Design review of the part built by this model. Coordinates are the model's own, in mm. Face numbers are marked on the shaded views. Coordinates: 2 decimals unless noted, no trailing zeros. Loops run counter-clockwise (first coordinate to the right, second up) from the corner with the lowest first, then second, coordinate; pieces in that order, holes last. Notation, with made-up numbers: (54.25, 68) -> (61.25, 68) arc R18 cw to (61.25, 98) -> close; hole circle Ø3 at (80, 89.5). An arc over 180 degrees is marked (long way). Use CSV: the item, a comma, the result in double quotes.
```python
from build123d import *

# Parameters (mm, degrees)
EXTRUDE_1_DEPTH             = 20
SKETCH_2_R                  = 15
CUT_EXTRUDE_1_DEPTH         = 21
CUT_EXTRUDE_2_DEPTH         = 5
HOLE_WIZARD_M6_1_D          = 5
HOLE_WIZARD_M6_1_DEPTH      = 15
HOLE_WIZARD_M6_1_TIP        = 1.502151548
HOLE_WIZARD_M6_2_AT_2_COUNT = 2
HOLE_WIZARD_M6_2_AT_2_PITCH = 40
MM_1_D                      = 12
MM_1_DEPTH                  = 2
MM_1_TIP                    = 3.605163714
SKETCH_19_W                 = 298.256507651
SKETCH_19_H                 = 73.483487392
SKETCH_19_W_2               = 296.09522861
CUT_EXTRUDE_3_DEPTH         = 21


with BuildPart() as part:
    # 草图1 → 凸台-拉伸1 (new body)
    with BuildSketch(Plane.XY):
        Polygon((-580, 85), (-600, 65), (-600, -65), (-580, -85), (580, -85), (600, -65), (600, 65), (580, 85), align=None)
    extrude(amount=EXTRUDE_1_DEPTH)

    # 草图2 → 切除-拉伸1 (cut, through all)
    with BuildSketch(Plane.XY.offset(20)):
        with Locations((540, 0)):
            Circle(SKETCH_2_R)
    extrude(amount=-CUT_EXTRUDE_1_DEPTH, mode=Mode.SUBTRACT)

    # 草图3 → 切除-拉伸2 (cut)
    with BuildSketch(Plane.XY.offset(20)):
        with BuildLine():
            Line((-800, -60), (-405, -60))
            ThreePointArc((-405, -60), (-401.464466094, -58.535533906), (-400, -55))
            Line((-400, -55), (-400, 55))
            ThreePointArc((-400, 55), (-401.464466094, 58.535533906), (-405, 60))
            Line((-405, 60), (-800, 60))
            Line((-800, 60), (-800, -60))
        make_face()
    extrude(amount=-CUT_EXTRUDE_2_DEPTH, mode=Mode.SUBTRACT)

    # M6 螺纹孔1
    with Locations(Plane(origin=(-390, 25, 20), x_dir=(1, 0, 0), z_dir=(0, 0, 1))):
        with Locations((0, 0), (0, -50)):
            Hole(HOLE_WIZARD_M6_1_D / 2, depth=HOLE_WIZARD_M6_1_DEPTH)
            with Locations((0, 0, -(HOLE_WIZARD_M6_1_DEPTH + HOLE_WIZARD_M6_1_TIP / 2))):  # 118° drill point
                Cone(0, HOLE_WIZARD_M6_1_D / 2, HOLE_WIZARD_M6_1_TIP, mode=Mode.SUBTRACT)

    # 草图16 → M6 螺纹孔2 (revolve, cut)
    with BuildSketch(Plane(origin=(400, 60, 20), x_dir=(0, -1, 0), z_dir=(1, 0, 0))):
        Polygon((0, 0), (0, 16.502151548), (2.5, 15), (2.5, 0), align=None)
    hole_wizard_m6_2 = revolve(axis=Axis((400, 60, 26.35), (0, 0, -1)), mode=Mode.SUBTRACT)

    # M6 螺纹孔2 at 2: M6 螺纹孔2 ×2
    with Locations(*[(i * HOLE_WIZARD_M6_2_AT_2_PITCH, 0, 0) for i in range(1, HOLE_WIZARD_M6_2_AT_2_COUNT)]):
        add(hole_wizard_m6_2, mode=Mode.SUBTRACT)

    # 镜向2: M6 螺纹孔2 across plane
    add(hole_wizard_m6_2.mirror(Plane.ZX), mode=Mode.SUBTRACT)

    # 镜向2 copy 1 sketch → 镜向2 copy 1 (revolve, cut)
    with BuildSketch(Plane(origin=(440, -60, 20), x_dir=(0, 1, 0), z_dir=(1, 0, 0))):
        Polygon((0, 0), (0, -16.502151548), (2.5, -15), (2.5, 0), align=None)
    revolve(axis=Axis((440, -60, 26.35), (0, 0, 1)), mode=Mode.SUBTRACT)

    # 大小mm 暗销孔1
    with Locations(Plane(origin=(0, 0, 0), x_dir=(-1, 0, 0), z_dir=(0, 0, -1))):
        with Locations((-250, 65), (250, 65), (250, -65), (-250, -65)):
            Hole(MM_1_D / 2, depth=MM_1_DEPTH)
            with Locations((0, 0, -(MM_1_DEPTH + MM_1_TIP / 2))):  # 118° drill point
                Cone(0, MM_1_D / 2, MM_1_TIP, mode=Mode.SUBTRACT)

    # 草图19 → 切除-拉伸3 (cut, through all)
    with BuildSketch(Plane.XY.offset(20)):
        with Locations((-182.687664533, 0)):
            Rectangle(SKETCH_19_W, SKETCH_19_H)
        with Locations((286.309887354, 0)):
            Rectangle(SKETCH_19_W_2, SKETCH_19_H)
    extrude(amount=-CUT_EXTRUDE_3_DEPTH, mode=Mode.SUBTRACT)


solid = part.part
```
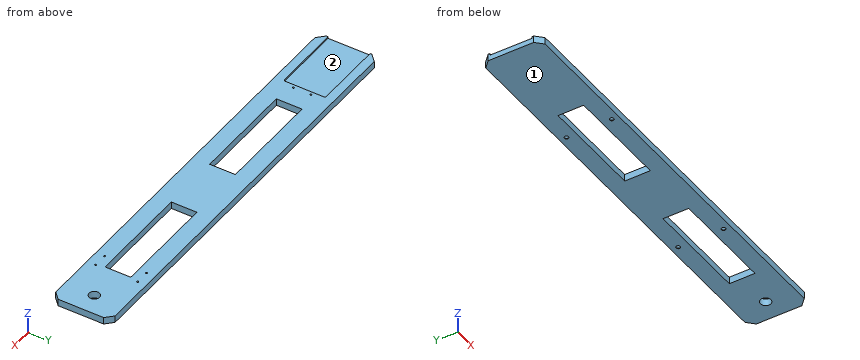
Item 1: Clearance check with a flat-ended pin moving along its axis: pin 1 (3 mm diameter, centred on x = 400, y = -60, fed in from +Z). State where the tip first meets the part, or that it passes through.
Checked values:
pin 1,"z = 4.4"
Item 2: To check wall thickness, follow line 1 along X through (y, z) = (65, 0.9); line 2 along Y through (x, z) = (250, 0.9); line 3 along X through (y, z) = (60, 14). State the ranges of each line that lie inside material, in increasing order.
Checked values:
line 1,"-600 to -256, -244 to 244, 256 to 600"
line 2,"-85 to -71, -59 to -36.74, 36.74 to 59, 71 to 85"
line 3,"-600 to 397.5, 402.5 to 437.5, 442.5 to 600"
Item 3: Draft analysis for pull direction Y (two halves, no side actions). For the marked faces 1 and 2, state which applies: pulls with the +Y half, pulls with the -Y half, needs draft (parallel to the pull), parting line crosses it, or undercut.
Checked values:
face 1,"needs draft"
face 2,"undercut"
Item 4: Add section A-A (x = -83). Give the boundary of the cut face in (y, z).
Checked values:
outline,"(-85, 0) -> (-36.74, 0) -> (-36.74, 20) -> (-85, 20) -> close; (36.74, 0) -> (85, 0) -> (85, 20) -> (36.74, 20) -> close"
Item 5: Add section B-B (x = 540). Give the boundary of the cut face in (y, z).
Checked values:
outline,"(-85, 0) -> (-15, 0) -> (-15, 20) -> (-85, 20) -> close; (15, 0) -> (85, 0) -> (85, 20) -> (15, 20) -> close"
